CAD build for the part. Positions are in the model's coordinates, mm. Face numbers are marked on the shaded views. A direction names the side the tool comes from. Coordinates: 2 decimals unless noted, no trailing zeros. Answer in a Markdown table with one row per item. Add a question column.
Q1. 3-axis set-ups, long thin cutter, end or side, ignore diameter. For the marked faces 1 and 2: which of +Z, -Z, +X, -X, +Y, -Y reach the whole face in a straight line?
Q2. Pin check, flat tips, straight feed: pin 1 (4 mm diameter, centred on x = -7.5, y = 7, fed in from -Z); pin 2 (1.2 mm diameter, centred on x = 11.5, z = 56, fed in from +Y); pin 3 (1.7 mm diameter, centred on y = -11.5, z = 57.5, fed in from +X); pin 4 (1 mm diameter, centred on x = -4, z = 39, fed in from +Y). Stop position of each tip, or through.
Q3. Drill centre lines: line 1 along Y through (x, z) = (0, 53); line 2 along Z through (x, y) = (-2, 6); line 3 along X through (y, z) = (2, 57.5). Where is each one in solid material? Low to high. Write a range as from..to.
Q4. Two-plate mould, pull along Y, no slides. Class the marked faces 3, 4 and 5: +Y half, -Y half, draft (parallel to the pull), parting line (faces both ways), or undercut.
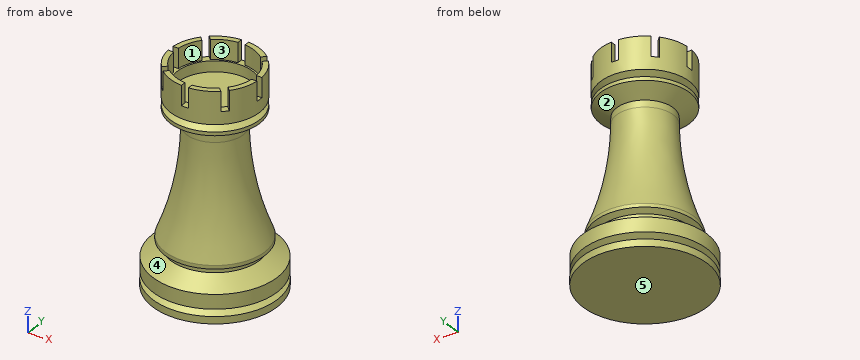
```python
from build123d import *

# Parameters (mm, degrees)
F3_DEPTH = 27
F4_R     = 10.5
F5_DEPTH = 3


with BuildPart() as f1:
    # F0 (on Front) → F1 (revolve)
    with BuildSketch(Plane.XZ):
        with BuildLine():
            Line((0, 6), (0, 0))
            Line((0, 0), (17.5, 0))
            Line((17.5, 0), (17.5, 2))
            Line((17.5, 2), (15.767949, 3))
            Line((15.767949, 3), (17.445428, 3.968493))
            Line((17.445428, 3.968493), (17.445428, 7.968493))
            Line((17.445428, 7.968493), (12.445428, 10.855244))
            Line((12.445428, 10.855244), (12.445428, 11.855244))
            Line((12.445428, 11.855244), (14, 12.752777))
            Line((14, 12.752777), (14, 13.752777))
            ThreePointArc((14, 13.752777), (9.586573, 28.322839), (7.982154, 43.461892))
            Line((7.982154, 43.461892), (7.960461, 45.379096))
            Line((7.960461, 45.379096), (12.5, 48))
            Line((12.5, 48), (12.5, 49))
            Line((12.5, 49), (10.767949, 50))
            Line((10.767949, 50), (12.5, 51))
            Line((12.5, 51), (12.5, 60))
            Line((12.5, 60), (11, 60))
            Line((11, 60), (11, 54.5))
            Line((11, 54.5), (0, 54.5))
            Line((0, 54.5), (0, 6))
        make_face()
    revolve(axis=Axis((0, 0, 30), (0, 0, 1)))

    # F2 (on face) → F3 (cut)
    with BuildSketch(Plane.XY.offset(54.5)):
        Polygon((1, 0), (0, 0), (-0.707107, 0.707107), (-1, 0.414214), (-1, -0.414214), (-0.414214, -1), (0.414214, -1), (1, -1), (1, -0.414214), align=None)
        Polygon((2.414214, 1), (1.414214, 0), (33.121221, 0), (33.121221, 1), align=None)
        Polygon((33.121221, 0), (1.414214, 0), (2.414214, -1), (33.121221, -1), align=None)
        Polygon((-1, 2.414214), (0, 1.414214), (0, 23.9831), (-1, 23.9831), align=None)
        Polygon((0, 23.9831), (0, 1.414214), (1, 2.414214), (1, 23.9831), align=None)
        Polygon((21.433732, 21.433732), (1, 1), (2.414214, 1), (22.140839, 20.726625), align=None)
        Polygon((1, 2.414214), (1, 1), (21.433732, 21.433732), (20.726625, 22.140839), align=None)
        Polygon((-18.999232, 18.999232), (-1, 1), (-1, 2.414214), (-18.31192, 19.726133), align=None)
        Polygon((-2.414214, 1), (-1, 1), (-18.999232, 18.999232), (-19.686545, 18.272332), align=None)
        Polygon((21.433732, -20.019518), (2.414214, -1), (1, -1), (1, -2.414214), (20.019518, -21.433732), align=None)
        Polygon((-2.414214, -1), (-1.414214, 0), (-2.414214, 1), (-22.418227, 1), (-22.418227, -1), align=None)
        Polygon((1, -22.243075), (1, -2.414214), (0, -1.414214), (-1, -2.414214), (-1, -22.243075), align=None)
        Polygon((-1, -2.414214), (-1, -1), (-2.414214, -1), (-23.888705, -22.474491), (-22.474491, -23.888705), align=None)
    extrude(amount=F3_DEPTH, mode=Mode.SUBTRACT)

    # F4 (on face) → F5 (cut)
    with BuildSketch(Plane.XY.offset(54.5)):
        Circle(F4_R)
    extrude(amount=-F5_DEPTH, mode=Mode.SUBTRACT)


solid = f1.part
```
Checked values:
| question | item | result |
|---|---|---|
| 1 | face 1 | +Z |
| 1 | face 2 | none |
| 2 | pin 1 | stops at z = 0 |
| 2 | pin 2 | stops at y = 6.12 |
| 2 | pin 3 | stops at x = 6.54 |
| 2 | pin 4 | stops at y = 7.37 |
| 3 | line 1 | y = -12.5..-10.5, 10.5..12.5 |
| 3 | line 2 | z = 0..51.5 |
| 3 | line 3 | x = -12.34..-10.82, 10.82..12.34 |
| 4 | face 3 | undercut |
| 4 | face 4 | parting line |
| 4 | face 5 | draft |
